```python
from build123d import *

# Parameters (mm, degrees)
SKETCH_1_R          = 22.5
EXTRUDE_1_DEPTH     = 13.4
SKETCH_5_R          = 21.001588026
CUT_EXTRUDE_1_DEPTH = 11
SKETCH_6_R          = 8
CUT_EXTRUDE_2_DEPTH = 3
EXTRUDE_START       = -9
EXTRUDE_6_DEPTH     = 9
EXTRUDE_7_DEPTH     = 1
EXTRUDE_8_DEPTH     = 7
CHAMFER_1_SIZE      = 0.5
SKETCH_13_R         = 9.5
CUT_EXTRUDE_4_DEPTH = 2
EXTRUDE_10_DEPTH    = 13.4


with BuildPart() as part:
    # Эскиз1 → Бобышка-Вытянуть1 (new body)
    with BuildSketch(Plane(origin=(0, 0, 0), x_dir=(1, 0, 0), z_dir=(0, 1, 0))):
        with Locations(Location((0, 0, 0), (0, 0, 270))):
            Circle(SKETCH_1_R)
    extrude(amount=EXTRUDE_1_DEPTH)

    # Эскиз5 → Вырез-Вытянуть1 (cut)
    with BuildSketch(Plane(origin=(0, 13.4, 0), x_dir=(1, 0, 0), z_dir=(0, 1, 0))):
        with Locations(Location((0, 0, 0), (0, 0, 270))):
            Circle(SKETCH_5_R)
    extrude(amount=-CUT_EXTRUDE_1_DEPTH, mode=Mode.SUBTRACT)

    # Эскиз6 → Вырез-Вытянуть2 (cut)
    with BuildSketch(Plane(origin=(0, 0, 0), x_dir=(-1, 0, 0), z_dir=(0, -1, 0))):
        with Locations(Location((0, 0, 0), (0, 0, 90))):
            Circle(SKETCH_6_R)
    extrude(amount=-CUT_EXTRUDE_2_DEPTH, mode=Mode.SUBTRACT)

    # Эскиз8 → Бобышка-Вытянуть6 (add)
    with BuildSketch(Plane(origin=(0, 13.4, 0), x_dir=(1, 0, 0), z_dir=(0, 1, 0)).offset(EXTRUDE_START)):
        with BuildLine():
            Line((7.917321695, 23.713203436), (6.638578465, 21.498355192))
            ThreePointArc((6.638578465, 21.498355192), (11.25, 19.485571585), (15.298832503, 16.498355192))
            Line((15.298832503, 16.498355192), (16.577575733, 18.713203436))
            ThreePointArc((16.577575733, 18.713203436), (12.5, 21.650635095), (7.917321695, 23.713203436))
        make_face()
        with BuildLine():
            Line((-7.917321695, -23.713203436), (-6.638578465, -21.498355192))
            ThreePointArc((-6.638578465, -21.498355192), (-11.25, -19.485571585), (-15.298832503, -16.498355192))
            Line((-15.298832503, -16.498355192), (-16.577575733, -18.713203436))
            ThreePointArc((-16.577575733, -18.713203436), (-12.5, -21.650635095), (-7.917321695, -23.713203436))
        make_face()
    extrude(amount=EXTRUDE_6_DEPTH)

    # Эскиз9 → Бобышка-Вытянуть7 (add)
    with BuildSketch(Plane(origin=(0, 13.4, 0), x_dir=(1, 0, 0), z_dir=(0, 1, 0))):
        Polygon((8.069392034, 22.476596989), (7.869392034, 22.130186827), (15.230607966, 17.880186827), (15.430607966, 18.226596989), align=None)
        Polygon((-8.069392034, -22.476596989), (-15.430607966, -18.226596989), (-15.230607966, -17.880186827), (-7.869392034, -22.130186827), align=None)
    extrude(amount=EXTRUDE_7_DEPTH)

    # Эскиз10 → Бобышка-Вытянуть8 (add)
    with BuildSketch(Plane(origin=(0, 14.4, 0), x_dir=(1, 0, 0), z_dir=(0, 1, 0))):
        Polygon((10.580865705, 21.026596989), (10.380865705, 20.680186827), (12.719134295, 19.330186827), (12.919134295, 19.676596989), align=None)
        Polygon((-10.580865705, -21.026596989), (-12.919134295, -19.676596989), (-12.719134295, -19.330186827), (-10.380865705, -20.680186827), align=None)
    extrude(amount=EXTRUDE_8_DEPTH)

    # Фаска1
    chamfer_1_edges = [part.edges().sort_by_distance(p)[0] for p in [
        (10.480865705, 21.4, -20.853391908),
        (12.819134295, 21.4, -19.503391908),
        (-10.480865705, 21.4, 20.853391908),
        (-12.819134295, 21.4, 19.503391908),
    ]]
    chamfer(chamfer_1_edges, length=CHAMFER_1_SIZE)

    # Эскиз11 → Повернуть1 (revolve)
    with BuildSketch(Plane(origin=(0, 0, 0), x_dir=(0, 0, -1), z_dir=(1, 0, 0))):
        Polygon((20.5, 2.4), (17.5, 2.4), (5, 9.616878365), (5, 10.9), (15.75, 10.9), (15.75, 11.4), (0, 11.4), (0, 10.9), (4.5, 10.9), (4.5, 9.32820323), (17.366025404, 1.9), (20.5, 1.9), align=None)
    revolve(axis=Axis((0, 0, 0), (0, 1, 0)))

    # Эскиз13 → Вырез-Вытянуть4 (cut)
    with BuildSketch(Plane.XZ):
        with Locations(Location((0, 0, 0), (0, 0, 270))):
            Circle(SKETCH_13_R)
    extrude(amount=-CUT_EXTRUDE_4_DEPTH, mode=Mode.SUBTRACT)

    # Эскиз15 → Бобышка-Вытянуть10 (add)
    with BuildSketch(Plane.XZ):
        with BuildLine():
            Line((-21.937410968, 5), (-22.75, 5))
            Line((-22.75, 5), (-22.75, -5))
            Line((-22.75, -5), (-21.937410968, -5))
            ThreePointArc((-21.937410968, -5), (-22.5, 0), (-21.937410968, 5))
        make_face()
        with BuildLine():
            Line((22.75, 5), (22.75, -5))
            Line((22.75, -5), (21.937410968, -5))
            ThreePointArc((21.937410968, -5), (22.5, 0), (21.937410968, 5))
            Line((21.937410968, 5), (22.75, 5))
        make_face()
    extrude(amount=-EXTRUDE_10_DEPTH)


solid = part.part
```
Geometry check sheet. Reference: the model listing, model coordinates, mm. A direction names the side the tool comes from. Coordinates: 2 decimals unless noted, no trailing zeros. Loops run counter-clockwise (first coordinate to the right, second up) from the corner with the lowest first, then second, coordinate; pieces in that order, holes last. Notation, with made-up numbers: (-25, 77.25) - (9, 77.25) arc R10 ccw to (9, 88.25) - close; hole circle Ø4 at (16.5, -36). An arc over 180 degrees is marked (long way). One line per item, written item: value. Start each with the question number.
(1) Tool access check on faces 5 (the flat face through (-7, 2, 4.3)), 6 (the flat face through (7.287, 8.837, -22.621)), 7 (the flat face through (0, 11.4, 0)). Record the directions out of +Z, -Z, +X, -X, +Y, -Y that give a thin tool (end or side, any length) a straight path to the whole face; none if there is none.
(2) Mould release check, pull along X, two halves, no side actions. Record for faces 1 (the flat face through (-14.1, 14.4, 18.8)), 2 (the flat face through (8, 2.4, 3)), 3 (the cylindrical face through (17.71, 7.98, 11.29)), 4 (the cylindrical face through (12.561, 8.837, -21.615)): released by +X, released by -X, zero draft, split by the parting line, or undercut.
(3) Cross-section at B-B on y = 16. Enter the section's corners in (x, z).
(4) Depth check by flat-ended pin: P1, Ø2, axis at x = -15, y = 7.5, coming from the -Z side; P2, Ø1.4, axis at x = -9.5, z = 22, coming from the +Y side; P3, Ø8, axis at x = 0, z = 0, coming from the -Y side. Enter the tip coordinate at first touch or a pass-through.
(5) Material ranges on line 1 (X direction, y = 10.3, z = 0); line 2 (X direction, y = 4.5, z = -9); line 3 (Y direction, x = 8.5, z = -7.5), recorded low to high. Write a range as [from, to].
(6) Cross-section at A-A on y = 6. Enter the section's corners in (x, z), plus the area to 3 significant figures.
Results below:
1. face 5: -Y
1. face 6: -Z, +Y, -Y
1. face 7: +Y
2. face 1: zero draft
2. face 2: undercut
2. face 3: undercut
2. face 4: released by +X
3. outline: (-12.92, 19.68) - (-12.72, 19.33) - (-10.38, 20.68) - (-10.58, 21.03) - close; (10.38, -20.68) - (10.58, -21.03) - (12.92, -19.68) - (12.72, -19.33) - close
4. P1: stops at z = -17.61
4. P2: stops at y = 14.4
4. P3: stops at y = 10.9
5. line 1: x = [-22.75, -21], [-5, -4.5], [4.5, 5], [21, 22.75]
5. line 2: x = [-20.62, -18.98], [-10.54, -9.19], [9.19, 10.54], [18.98, 20.62]
5. line 3: y = [0, 2.4], [5.38, 5.96], [10.9, 11.4]
6. outline: (-22.75, -5) - (-21.94, -5) arc R22.5 ccw to (6.64, -21.5) - (7.92, -23.71) arc R25 ccw to (16.58, -18.71) - (15.3, -16.5) arc R22.5 ccw to (21.94, -5) - (22.75, -5) - (22.75, 5) - (21.94, 5) arc R22.5 ccw to (-6.64, 21.5) - (-7.92, 23.71) arc R25 ccw to (-16.58, 18.71) - (-15.3, 16.5) arc R22.5 ccw to (-21.94, 5) - (-22.75, 5) - close; circle Ø22.53 at (0, 0); hole circle Ø42 at (0, 0); hole circle Ø20.53 at (0, 0)
6. area: 332 mm2
